from build123d import *

# Parameters (mm, degrees)
BOSS_EXTRUDE1_DEPTH            = 4
SKETCH3_W                      = 59.68
SKETCH3_H                      = 8
BOSS_EXTRUDE2_DEPTH            = 5.46
SKETCH5_W                      = 2.16
SKETCH5_H                      = 59.704316385
CUT_EXTRUDE2_DEPTH             = 9
CUT_EXTRUDE3_DEPTH             = 9
CBORE_FOR_M3_SHCS2_D           = 3.4
CBORE_FOR_M3_SHCS2_CBORE_D     = 6.5
CBORE_FOR_M3_SHCS2_CBORE_DEPTH = 3
M2X0_4_TAPPED_HOLE1_D          = 1.6
M2X0_4_TAPPED_HOLE1_DEPTH      = 7
M2X0_4_TAPPED_HOLE1_TIP        = 0.480688495
CUT_EXTRUDE4_DEPTH             = 9
SKETCH22_R                     = 1.5
CUT_EXTRUDE6_DEPTH             = 5.5
M3X0_5_TAPPED_HOLE2_D          = 2.5
M3X0_5_TAPPED_HOLE2_DEPTH      = 8.5
M3X0_5_TAPPED_HOLE2_TIP        = 0.751075774


with BuildPart() as part:
    # Sketch2 → Boss-Extrude1 (new body, symmetric)
    with BuildSketch(Plane.XY):
        Polygon((-8.360559535, 17.409242356), (51.319440465, 17.409242356), (51.319440465, 71.653558741), (36.009440465, 71.653558741), (43.084036895, 64.586021309), (-1.285963105, 20.171704924), (-8.360559535, 27.239242356), align=None)
    extrude(amount=BOSS_EXTRUDE1_DEPTH, both=True)

    # Sketch3 → Boss-Extrude2 (add)
    with BuildSketch(Plane.XZ.offset(-17.409242356)):
        with Locations((21.479440465, 0)):
            Rectangle(SKETCH3_W, SKETCH3_H)
    extrude(amount=BOSS_EXTRUDE2_DEPTH)

    # Sketch5 → Cut-Extrude2 (cut, through all)
    with BuildSketch(Plane.XY.offset(4)):
        with Locations((50.239440465, 41.801400548)):
            Rectangle(SKETCH5_W, SKETCH5_H)
    extrude(amount=-CUT_EXTRUDE2_DEPTH, mode=Mode.SUBTRACT)

    # Sketch9 → Cut-Extrude3 (cut, through all)
    with BuildSketch(Plane.XY.offset(4)):
        Polygon((36.009440465, 71.653558741), (49.159440465, 58.503558741), (49.159440465, 71.653558741), align=None)
    extrude(amount=-CUT_EXTRUDE3_DEPTH, mode=Mode.SUBTRACT)

    # CBORE for M3 SHCS2 (through all)
    with Locations(Plane(origin=(49.159440465, 0, 0), x_dir=(0, 0, -1), z_dir=(1, 0, 0))):
        with Locations((0, 48.503558741)):
            CounterBoreHole(CBORE_FOR_M3_SHCS2_D / 2, CBORE_FOR_M3_SHCS2_CBORE_D / 2, CBORE_FOR_M3_SHCS2_CBORE_DEPTH)

    # M2x0.4 Tapped Hole1
    with Locations(Plane.XY.offset(4)):
        with Locations((30.839440465, 13.949242356), (40.839440465, 13.949242356)):
            Hole(M2X0_4_TAPPED_HOLE1_D / 2, depth=M2X0_4_TAPPED_HOLE1_DEPTH)
            with Locations((0, 0, -(M2X0_4_TAPPED_HOLE1_DEPTH + M2X0_4_TAPPED_HOLE1_TIP / 2))):  # 118° drill point
                Cone(0, M2X0_4_TAPPED_HOLE1_D / 2, M2X0_4_TAPPED_HOLE1_TIP, mode=Mode.SUBTRACT)

    # Sketch20 → Cut-Extrude4 (cut, through all)
    with BuildSketch(Plane.XY.offset(4)):
        Polygon((-1.285963105, 20.171704924), (-1.285963105, 11.949242356), (-8.360559535, 11.949242356), (-8.360559535, 27.239242356), align=None)
    extrude(amount=-CUT_EXTRUDE4_DEPTH, mode=Mode.SUBTRACT)

    # Sketch22 → Cut-Extrude6 (cut)
    with BuildSketch(Plane(origin=(-10.729470873, 10.71876506, 0), x_dir=(0, 0, 1), z_dir=(-0.707459643, 0.706753743, 0))):
        with Locations((0, 23.361807925)):
            Circle(SKETCH22_R)
    extrude(amount=-CUT_EXTRUDE6_DEPTH, mode=Mode.SUBTRACT)

    # M3x0.5 Tapped Hole2
    with Locations(Plane.ZY.offset(1.285963105)):
        with Locations((0, 15.949242356)):
            Hole(M3X0_5_TAPPED_HOLE2_D / 2, depth=M3X0_5_TAPPED_HOLE2_DEPTH)
            with Locations((0, 0, -(M3X0_5_TAPPED_HOLE2_DEPTH + M3X0_5_TAPPED_HOLE2_TIP / 2))):  # 118° drill point
                Cone(0, M3X0_5_TAPPED_HOLE2_D / 2, M3X0_5_TAPPED_HOLE2_TIP, mode=Mode.SUBTRACT)


solid = part.part
Can you work these out from the model? Positions are in its coordinate system, mm. A direction names the side the tool comes from. Round coordinates to 2 decimals unless told otherwise and drop trailing zeros. Write each loop counter-clockwise with the first axis right and the second up, starting at its lowest first coordinate (ties: lowest second). Pieces come first, ordered by that corner, then holes. Notation, with made-up numbers: (-36, -14.5) - (5, -14.5) arc R28 ccw to (5, 22.5) - close; hole circle Ø2 at (31, 33.25). An arc over 180 degrees is marked (long way). Write each question's results on one line, items separated by ' | '. Start each with the question number.
1) We'd pull the mould along Z, two halves only. Please class faces 6 (the cylindrical face through (30.076, 14.19, 0.451)), 7 (the cylindrical face through (8.75, 26.38, -0.2)), 8 (the conical face through (40.809, 13.814, -3.397)), 9 (the cylindrical face through (47.68, 51.726, 0.423)): released by +Z, released by -Z, zero draft, split by the parting line, or undercut.
2) Suppose I cut it at D-D (y = 36.5). List the corners of the cut face in (x, z) for me.
3) Which directions (+Z, -Z, +X, -X, +Y, -Y) give clear straight access to the entire face, cutting with the end or side of a thin tool? Please do faces 1 (the flat face through (-1.286, 17, 1)), 2 (the flat face through (46.159, 47.1, -1.4)), 3 (the cylindrical face through (3.024, 17.003, -0.672)), 4 (the cylindrical face through (40.409, 14.624, 0.451)), 5 (the flat face through (9.687, 23.374, -0.021)).
4) For pin 1 Ø3 at (x, z) = (25.5, 0) entering from +Y; pin 2 Ø1.3 at (x, y) = (40.84, 13.95) entering from +Z; pin 3 Ø2 at (y, z) = (49.5, 0.5) entering from +X, each with a flat end and sliding along its axis, tell me the tip position at first contact or that it passes through.
5) Suppose I cut it at B-B (x = 39). List the corners of the cut face in (y, z) for me, and give its area (3 significant figures).
6) Suppose I cut it at A-A (y = 47.5). List the corners of the cut face in (x, z) for me, and give its area (3 significant figures).
7) Suppose I cut it at C-C (x = 22). List the corners of the cut face in (y, z) for me, and give its area (3 significant figures).
8) Please list where these lines run through material, in increasing order: line 1 (Y direction, x = 30.5, z = 1); line 2 (Y direction, x = 46.5, z = -1.25); line 3 (Y direction, x = 1.75, z = 0).
Here are the results:
1) face 6: zero draft | face 7: undercut | face 8: released by +Z | face 9: undercut
2) outline: (15.03, -4) - (49.16, -4) - (49.16, 4) - (15.03, 4) - close
3) face 1: +Z, -Z, -X, +Y, -Y | face 2: +X | face 3: -X | face 4: +Z | face 5: none
4) pin 1: stops at y = 47.53 | pin 2: stops at z = -3.09 | pin 3: stops at x = 46.16
5) outline: (11.95, -4) - (60.5, -4) - (60.5, 4) - (11.95, 4) - close; hole circle Ø3.4 at (48.5, 0) | area: 379 mm2
6) outline: (26.02, -4) - (49.16, -4) - (49.16, -3.09) - (46.16, -3.09) - (46.16, -1.37) - (26.02, -1.37) - close; (26.02, 1.37) - (46.16, 1.37) - (46.16, 3.09) - (49.16, 3.09) - (49.16, 4) - (26.02, 4) - close | area: 111 mm2
7) outline: (11.95, -4) - (43.48, -4) - (43.48, 4) - (11.95, 4) - close | area: 252 mm2
8) line 1: y = 11.95 to 13.22, 14.67 to 47.13, 49.88 to 51.99 | line 2: y = 11.95 to 45.5, 51.5 to 61.16 | line 3: y = 11.95 to 14.7, 17.2 to 23.21
